Read the model definition and answer for the solid it produces. Units are mm, in the model's axes. A direction names the side the tool comes from. Give positions to 0.01 mm unless a question says otherwise; leave off trailing zeros. Order: outer loops, then holes, each group sorted by start corner. A loop starts at its lowest first (then second) coordinate and runs counter-clockwise, first axis right, second up. Notation, with made-up numbers: (-12, 57.25) -> (5, 57.25) arc R14 ccw to (5, 72.25) -> close; hole circle Ø2 at (11, 49.5). An arc over 180 degrees is marked (long way). Answer as CSV lines item,"result". Start each with the question number.
1) Find section A-A (x = 0). Determine the outline of the cut face in (y, z), and give its area (3 significant figures).
2) Find section C-C (x = 189). Determine the outline of the cut face in (y, z).
3) Straight lines are drawn through the part: L1, parallel to X at y = 3.95, z = 0; L2, parallel to X at y = 2.25, z = -2.5; L3, parallel to X at y = 3.45, z = -0.5. For each, find the intervals that lie inside material, in ascending order. Write a range as from..to.
4) Flat-ended cylindrical pins translate along their axes: pin 1 Ø1 at (y, z) = (4, 5) entering from -X; pin 2 Ø1.5 at (x, y) = (38, 3) entering from -Z; pin 3 Ø3 at (x, y) = (157, 0.5) entering from +Z. Find the tip coordinate at first contact, or state that the pin passes through.
5) The mould has two halves that part along X. Classify faces 1 (the face through (137, 2, -6)), 2 (the face through (60, 2, 9)), 3 (the face through (198.226, 2.535, 0.923)), 4 (the face through (210, 2, 0)): +X half, -X half, draft (parallel to the pull), parting line (faces both ways), or undercut.
6) Find section B-B (y = 3.5). Determine the outline of the cut face in (x, z).
7) For faces 5 (the face through (30, 2, 6)), 6 (the face through (30, 2, -6)), 7 (the face through (139, 2, 6)), determine the directions among +Z, -Z, +X, -X, +Y, -Y from which every point of the face is accessible in a straight line to the end or side of a thin tool.
```python
from build123d import *

# Parameters (mm, degrees)
BOSS_EXTRUDE1_DEPTH = 5
SKETCH2_R           = 5
SKETCH2_R_2         = 2
CUT_EXTRUDE1_DEPTH  = 211.252229477


with BuildPart() as part:
    # Sketch1 → Boss-Extrude1 (new body)
    with BuildSketch(Plane(origin=(0, 0, 0), x_dir=(1, 0, 0), z_dir=(0, 1, 0))):
        with BuildLine():
            Line((6.708203932, 6), (53.291796068, 6))
            ThreePointArc((53.291796068, 6), (60, 9), (66.708203932, 6))
            Line((66.708203932, 6), (210, 6))
            Line((210, 6), (210, -6))
            Line((210, -6), (66.708203932, -6))
            ThreePointArc((66.708203932, -6), (60, -9), (53.291796068, -6))
            Line((53.291796068, -6), (6.708203932, -6))
            ThreePointArc((6.708203932, -6), (-9, 0), (6.708203932, 6))
        make_face()
    extrude(amount=BOSS_EXTRUDE1_DEPTH)

    # Sketch2 → Cut-Extrude1 (cut, through all)
    with BuildSketch(Plane(origin=(0, 5, 0), x_dir=(1, 0, 0), z_dir=(0, 1, 0))):
        with Locations(Location((0, 0, 0), (0, 0, 270))):
            Circle(SKETCH2_R)
        with Locations(Location((60, 0, 0), (0, 0, 270))):
            Circle(SKETCH2_R)
        with Locations(Location((200, 0, 0), (0, 0, 270))):
            Circle(SKETCH2_R_2)
        with Locations(Location((180, 0, 0), (0, 0, 270))):
            Circle(SKETCH2_R_2)
    extrude(amount=-CUT_EXTRUDE1_DEPTH, mode=Mode.SUBTRACT)


solid = part.part
```
Findings below:
1,outline,"(0, -9) -> (5, -9) -> (5, -5) -> (0, -5) -> close; (0, 5) -> (5, 5) -> (5, 9) -> (0, 9) -> close"
1,area,"40.0 mm²"
2,outline,"(0, -6) -> (5, -6) -> (5, 6) -> (0, 6) -> close"
3,L1,"-9..-5, 5..55, 65..178, 182..198, 202..210"
3,L2,"-8.65..-4.33, 4.33..55.67, 64.33..210"
3,L3,"-8.99..-4.97, 4.97..55.03, 64.97..178.06, 181.94..198.06, 201.94..210"
4,pin 1,"x = -7.79"
4,pin 2,"z = -6"
4,pin 3,"z = 6"
5,face 1,"draft"
5,face 2,"undercut"
5,face 3,"undercut"
5,face 4,"+X half"
6,outline,"(6.71, -6) -> (53.29, -6) arc R9 ccw to (66.71, -6) -> (210, -6) -> (210, 6) -> (66.71, 6) arc R9 ccw to (53.29, 6) -> (6.71, 6) arc R9 ccw (long way) to start; hole circle Ø10 at (0, 0); hole circle Ø10 at (60, 0); hole circle Ø4 at (180, 0); hole circle Ø4 at (200, 0)"
7,face 5,"+Z, +Y, -Y"
7,face 6,"-Z, +Y, -Y"
7,face 7,"+Z, +X, +Y, -Y"
